```python
from build123d import *

# Parameters (mm, degrees)
SKIZZE3_R                       = 4
SCHNITT_LINEAR_AUSTRAGEN1_DEPTH = 20
SCHNITT_LINEAR_START            = -2
SKIZZE6_R                       = 5.15
SCHNITT_LINEAR_AUSTRAGEN2_DEPTH = 10.842719282


with BuildPart() as part:
    # Skizze1 → Rotation1 (revolve)
    with BuildSketch(Plane.XY):
        with BuildLine():
            Line((0, 12.5), (0, -12.5))
            ThreePointArc((0, -12.5), (-12.5, 0), (0, 12.5))
        make_face()
    revolve(axis=Axis((0, 27.42628623, 0), (0, -1, 0)))

    # Skizze3 → Schnitt-Linear austragen1 (cut, symmetric)
    with BuildSketch(Plane(origin=(0, 0, 0), x_dir=(1, 0, 0), z_dir=(0, 1, 0))):
        Circle(SKIZZE3_R)
    extrude(amount=SCHNITT_LINEAR_AUSTRAGEN1_DEPTH, both=True, mode=Mode.SUBTRACT)

    # Skizze5 → Rotation2 (revolve)
    with BuildSketch(Plane(origin=(0, 0, 0), x_dir=(0, 0, -1), z_dir=(1, 0, 0))):
        Polygon((-2.15, 0), (-2.15, 2), (-5, 3.712452764), (-5, 0), align=None)
    rotation2 = revolve(axis=Axis((0, 0, 0), (0, 1, 0)))

    # Spiegeln1: Rotation2 across plane
    add(rotation2.mirror(Plane.ZX))

    # Skizze6 → Schnitt-Linear austragen2 (cut, through all)
    with BuildSketch(Plane(origin=(0, 0, 0), x_dir=(1, 0, 0), z_dir=(0, 1, 0)).offset(SCHNITT_LINEAR_START)):
        Circle(SKIZZE6_R)
    extrude(amount=-SCHNITT_LINEAR_AUSTRAGEN2_DEPTH, mode=Mode.SUBTRACT)


solid = part.part
```
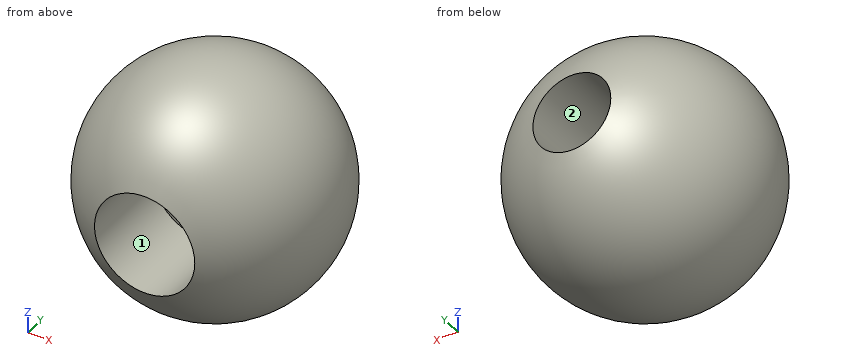
Geometry: final body of the model. Coordinates: model frame, mm. Face numbers are marked on the shaded views. Coordinates: 2 decimals unless noted, no trailing zeros. Write each loop counter-clockwise with the first axis right and the second up, starting at its lowest first coordinate (ties: lowest second). Pieces come first, ordered by that corner, then holes. Notation, with made-up numbers: M -32.5,-6.75 L 9.5,-6.75 A11 ccw 9.5,7.25 Z; hole C -38,40 d1. An arc over 180 degrees is marked long. Use CSV: the item, a comma, the result in double quotes. Start each with the question number.
1. Cut plane A-A on z = 0. Return the cut outline in (x, y), plus the area to 3 significant figures.
2. Mould query, pull axis X, two halves, no side actions, for the marked faces 1 and 2. Classes: pulls with the +X half, pulls with the -X half, needs draft (parallel to the pull), parting line crosses it, or undercut.
3. Cut plane C-C on x = -7. Return the cut outline in (y, z).
4. Ray query, probe 1 along X at (y, z) = (-8.5, -1); probe 2 along X at (y, z) = (10.25, 0); probe 3 along Z at (x, y) = (0, 7.25). Return the intervals inside material, ascending.
5. First-contact query: P1, Ø7, axis at x = 0, z = 0, coming from the +Y side; P2, Ø5.5, axis at x = 0, z = 0, coming from the -Y side; P3, Ø6, axis at x = -10, z = 2, coming from the -Y side. Flat tips, straight axial feed; report the tip coordinate or a pass-through.
6. Cut plane B-B on y = 0.5. Return the cut outline in (x, z).
7. Cut plane D-D on y = -9.5. Return the cut outline in (x, z).
Entries:
1,outline,"M -5.15,-11.39 L -5.15,-2 L -2.15,-2 L -2.15,2 L -4,3.11 L -4,11.84 A12.5 ccw Z; M 2.15,-2 L 5.15,-2 L 5.15,-11.39 A12.5 ccw 4,11.84 L 4,3.11 L 2.15,2 Z"
1,area,"289 mm²"
2,face 1,"undercut"
2,face 2,"undercut"
3,outline,"C 0,0 d20.71"
4,probe 1,"-9.11 to -5.05, 5.05 to 9.11"
4,probe 2,"-7.15 to -4, 4 to 7.15"
4,probe 3,"-10.18 to -4, 4 to 10.18"
5,P1,"y = 2.81"
5,P2,"y = -2"
5,P3,"y = -10.22"
6,outline,"C 0,0 d24.98; hole C 0,0 d4.3"
7,outline,"C 0,0 d16.25; hole C 0,0 d10.3"
